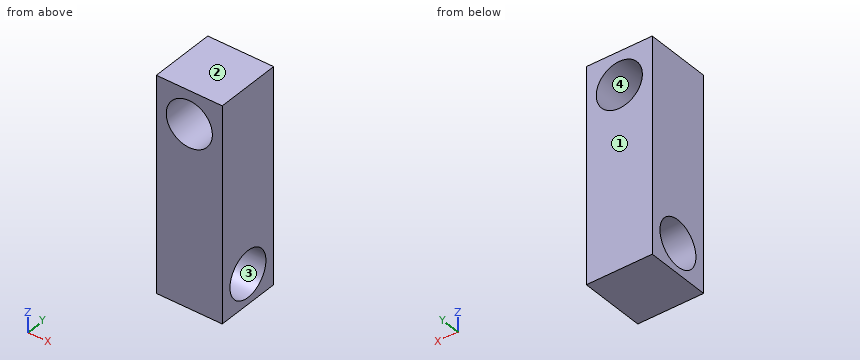
```python
from build123d import *

# Parameters (mm, degrees)
SZKIC1_W                    = 20
SZKIC1_H                    = 20
DODANIE_WYCI_GNI_CIE1_DEPTH = 65
SZKIC2_R                    = 7
WYTNIJ_WYCI_GNI_CIE1_DEPTH  = 50
SZKIC3_R                    = 7
WYTNIJ_WYCI_GNI_CIE2_DEPTH  = 50


with BuildPart() as part:
    # Szkic1 → Dodanie-wyciągnięcie1 (new body)
    with BuildSketch(Plane.XY):
        Rectangle(SZKIC1_W, SZKIC1_H)
    extrude(amount=DODANIE_WYCI_GNI_CIE1_DEPTH)

    # Szkic2 → Wytnij-wyciągnięcie1 (cut)
    with BuildSketch(Plane(origin=(10, 0, 0), x_dir=(0, 0, -1), z_dir=(1, 0, 0))):
        with Locations((-9.050144452, 0)):
            Circle(SZKIC2_R)
    extrude(amount=-WYTNIJ_WYCI_GNI_CIE1_DEPTH, mode=Mode.SUBTRACT)

    # Szkic3 → Wytnij-wyciągnięcie2 (cut)
    with BuildSketch(Plane(origin=(0, 10, 0), x_dir=(1, 0, 0), z_dir=(0, 1, 0))):
        with Locations(Location((0, -55, 0), (0, 0, 270))):
            Circle(SZKIC3_R)
    extrude(amount=-WYTNIJ_WYCI_GNI_CIE2_DEPTH, mode=Mode.SUBTRACT)


solid = part.part
```
The listing builds one solid part. Answer for the finished solid, in the listing's coordinates (mm). Face numbers are marked on the shaded views. Coordinates: 2 decimals unless noted, no trailing zeros. Write each loop counter-clockwise with the first axis right and the second up, starting at its lowest first coordinate (ties: lowest second). Pieces come first, ordered by that corner, then holes. Notation, with made-up numbers: (-34.75, 1.5) - (-24.75, 1.5) arc R29 ccw to (-24.75, 34.5) - close; hole circle Ø5 at (-3.75, -16.75). An arc over 180 degrees is marked (long way). Return JSON: item names as keys, results as strings. Group by question number.
Q1. The part is cut by section D-D on x = -7.75. Write down the section's boundary in (y, z).
Q2. Find the intervals of material crossed by line 1 along Z through (x, y) = (4.25, -3.5); line 2 along X through (y, z) = (1.25, 55); line 3 along Y through (x, z) = (3, 3.5), in increasing order. Write a range as [from, to].
Q3. The part is cut by section B-B on x = 0. Write down the section's boundary in (y, z).
Q4. For a pull along Z with two mould halves and no side action, classify the marked faces 1, 2, 3 and 4 as +Z half, -Z half, draft (parallel to the pull), parting line (faces both ways), or undercut.
Q5. The part is cut by section A-A on y = 0. Write down the section's boundary in (x, z).
Q6. The part is cut by section C-C on z = 55. Write down the section's boundary in (x, y).
Evaluation:
{
 "1": {"outline": "(-10, 0) - (10, 0) - (10, 65) - (-10, 65) - close; hole circle Ø14 at (0, 9.05)"},
 "2": {"line 1": "z = [0, 2.99], [15.11, 49.44], [60.56, 65]", "line 2": "x = [-10, -7], [7, 10]", "line 3": "y = [-10, -4.27], [4.27, 10]"},
 "3": {"outline": "(-10, 0) - (10, 0) - (10, 48) - (-10, 48) - close; (-10, 62) - (10, 62) - (10, 65) - (-10, 65) - close; hole circle Ø14 at (0, 9.05)"},
 "4": {"face 1": "draft", "face 2": "+Z half", "face 3": "undercut", "face 4": "undercut"},
 "5": {"outline": "(-10, 0) - (10, 0) - (10, 2.05) - (-10, 2.05) - close; (-10, 16.05) - (10, 16.05) - (10, 65) - (-10, 65) - close; hole circle Ø14 at (0, 55)"},
 "6": {"outline": "(-10, -10) - (-7, -10) - (-7, 10) - (-10, 10) - close; (7, -10) - (10, -10) - (10, 10) - (7, 10) - close"}
}
